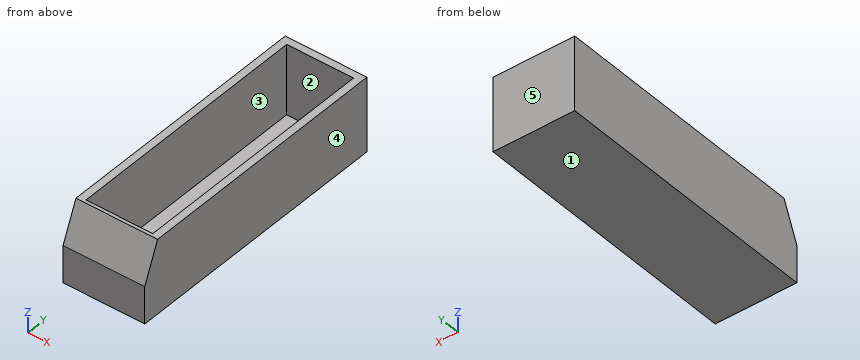
from build123d import *

# Parameters (mm, degrees)
F0_W     = 38.4
F0_H     = 129.5
F0_W_2   = 31.4
F0_H_2   = 111
F1_DEPTH = 2
F2_DEPTH = 35
F3_SIZE2 = 17.5
F3_SIZE  = 7.5
F4_SIZE2 = 32.99999
F4_SIZE  = 5.99999


# Not quite as in the source:
# - a fillet or chamfer is up to 0.001 mm smaller than in the source, because OpenCascade refuses the exact size


with BuildPart() as f1:
    # F0 (on Top) → F1 (new body)
    with BuildSketch(Plane.XY):
        with Locations((0, -5.75)):
            Rectangle(F0_W, F0_H)
        Rectangle(F0_W_2, F0_H_2, mode=Mode.SUBTRACT)
        Rectangle(F0_W_2, F0_H_2)
    extrude(amount=F1_DEPTH)

    # F0 (on Top) → F2 (join)
    with BuildSketch(Plane.XY):
        with Locations((0, -5.75)):
            Rectangle(F0_W, F0_H)
        Rectangle(F0_W_2, F0_H_2, mode=Mode.SUBTRACT)
    extrude(amount=F2_DEPTH)

    # F3
    f3_edges = [f1.edges().sort_by_distance(p)[0] for p in [
        (0, -70.5, 35),
    ]]
    f3_side = f1.faces().sort_by_distance((0, -69.149266, 35))[0]
    chamfer(f3_edges, length=F3_SIZE, length2=F3_SIZE2, reference=f3_side)

    # F4 (size 6 and 33 in the source; OpenCascade refuses exactly that, so slightly less here)
    f4_edges = [f1.edges().sort_by_distance(p)[0] for p in [
        (0, -55.5, 35),
    ]]
    f4_side = f1.faces().sort_by_distance((17.920994, -2, 35))[0]
    chamfer(f4_edges, length=F4_SIZE, length2=F4_SIZE2, reference=f4_side)


solid = f1.part
Geometry check sheet. Reference: the model listing, model coordinates, mm. Face numbers are marked on the shaded views. A direction names the side the tool comes from. Coordinates: 2 decimals unless noted, no trailing zeros. Order: outer loops, then holes, each group sorted by start corner. A loop starts at its lowest first (then second) coordinate and runs counter-clockwise, first axis right, second up. Notation, with made-up numbers: M 47.5,55.25 L 85.5,55.25 A35 cw 85.5,92.25 Z; hole C 15.25,87.5 d3. An arc over 180 degrees is marked long. Use CSV: the item, a comma, the result in double quotes.
Item 1: Gauge pin test, flat ends, axial feed: pin 1 Ø1.5 at (x, y) = (-1, -17) entering from +Z; pin 2 Ø4 at (x, z) = (2, 18.5) entering from -Y. Record the tip position at first contact, or that the pin passes through.
Returned:
pin 1,"stops at z = 2"
pin 2,"stops at y = -70.5"
Item 2: Tool access check on the marked faces 1 and 2. Record the directions out of +Z, -Z, +X, -X, +Y, -Y that give a thin tool (end or side, any length) a straight path to the whole face; none if there is none.
Returned:
face 1,"-Z, +X, -X, +Y, -Y"
face 2,"+Z"
Item 3: Mould release check, pull along X, two halves, no side actions. Record for the marked faces 3, 4 and 5: pulls with the +X half, pulls with the -X half, needs draft (parallel to the pull), parting line crosses it, or undercut.
Returned:
face 3,"undercut"
face 4,"pulls with the +X half"
face 5,"needs draft"
Item 4: Cross-section at C-C on y = 17. Record the cut outline in (x, z), then the cut area to 3 significant figures.
Returned:
outline,"M -19.2,0 L 19.2,0 L 19.2,35 L 15.7,35 L 15.7,2 L -15.7,2 L -15.7,35 L -19.2,35 Z"
area,"308 mm2"
Item 5: Cross-section at D-D on z = 27. Record the cut outline in (x, y), then the cut area to 3 significant figures.
Returned:
outline,"M -19.2,-66.43 L 19.2,-66.43 L 19.2,59 L -19.2,59 Z; hole M -15.7,-60.05 L 15.7,-60.05 L 15.7,55.5 L -15.7,55.5 Z"
area,"1,190 mm2"
Item 6: Thickness scan on line 1 along X through (y, z) = (-24.5, 11); line 2 along Z through (x, y) = (-6.5, 26); line 3 along Y through (x, z) = (-3, 27.5). Record the ranges inside material, lowest first.
Returned:
line 1,"x = -19.2 to -15.7, 15.7 to 19.2"
line 2,"z = 0 to 2"
line 3,"y = -66.21 to -60.14, 55.5 to 59"
